Build history of the part. All positions in model axes, mm. A direction names the side the tool comes from. Give positions to 0.01 mm unless a question says otherwise; leave off trailing zeros. Order: outer loops, then holes, each group sorted by start corner. A loop starts at its lowest first (then second) coordinate and runs counter-clockwise, first axis right, second up. Notation, with made-up numbers: (39.25, 64) -> (77.25, 64) arc R37 cw to (77.25, 100) -> close; hole circle Ø10 at (73, 73.25). An arc over 180 degrees is marked (long way). Use a Markdown table: item, result. Add a question column.
```python
from build123d import *

# Parameters (mm, degrees)
F0_R     = 3.175
F0_W     = 44.45
F0_H     = 76.2
F0_R_2   = 1.5875
F1_DEPTH = 3.175


with BuildPart() as f1:
    # F0 (on Top) → F1 (new body)
    with BuildSketch(Plane.XY):
        with BuildLine():
            ThreePointArc((16.728534, 58.82596), (-5.496466, 81.05096), (-27.721466, 58.82596))
            Line((-27.721466, 58.82596), (16.728534, 58.82596))
        make_face()
        with Locations((-5.496466, 69.93846)):
            Circle(F0_R, mode=Mode.SUBTRACT)
        with Locations((-5.496466, 20.72596)):
            Rectangle(F0_W, F0_H)
        with Locations((-5.496466, -4.67404)):
            Circle(F0_R_2, mode=Mode.SUBTRACT)
        with Locations((-5.496466, 8.02596)):
            Circle(F0_R_2, mode=Mode.SUBTRACT)
        with BuildLine():
            Line((-22.562091, -9.75404), (-22.562091, 51.20596))
            ThreePointArc((-22.562091, 51.20596), (-18.196466, 55.571585), (-13.830841, 51.20596))
            Line((-13.830841, 51.20596), (-13.830841, -9.75404))
            ThreePointArc((-13.830841, -9.75404), (-18.196466, -14.119665), (-22.562091, -9.75404))
        make_face(mode=Mode.SUBTRACT)
        with Locations((-5.496466, 46.12596)):
            Circle(F0_R_2, mode=Mode.SUBTRACT)
        with Locations((-5.496466, 20.72596)):
            Circle(F0_R_2, mode=Mode.SUBTRACT)
        with Locations((-5.496466, 33.42596)):
            Circle(F0_R_2, mode=Mode.SUBTRACT)
        with BuildLine():
            Line((2.837909, -9.75404), (2.837909, 51.20596))
            ThreePointArc((2.837909, 51.20596), (7.203534, 55.571585), (11.569159, 51.20596))
            Line((11.569159, 51.20596), (11.569159, -9.75404))
            ThreePointArc((11.569159, -9.75404), (7.203534, -14.119665), (2.837909, -9.75404))
        make_face(mode=Mode.SUBTRACT)
        with BuildLine():
            Line((16.728534, -17.37404), (-27.721466, -17.37404))
            ThreePointArc((-27.721466, -17.37404), (-5.496466, -39.59904), (16.728534, -17.37404))
        make_face()
        with Locations((-5.496466, -28.48654)):
            Circle(F0_R, mode=Mode.SUBTRACT)
    extrude(amount=F1_DEPTH)


solid = f1.part
```
(1) Mould opens along Y. For faces 3 (the face through (-5.008, 81.046, 1.565)), 4 (the face through (-5.841, 44.576, 1.565)), 5 (the face through (-27.721, 20, 2)) say: released by +Y, released by -Y, zero draft, split by the parting line, or undercut.
(2) Tool access for faces 1 (the face through (-18.29, 55.57, 1.57)), 2 (the face through (-1, 22, 3.175)): list every direction of +Z, -Z, +X, -X, +Y, -Y with a clear straight run to the whole face (end or side of a thin tool).
(3) Band-saw the part on C-C on x = -21.5. Give the cut face in (y, z) (3 decimals), plus the area to 3 significant figures.
(4) Band-saw the part on A-A on x = -5.5. State how many separate pieces and enclosed holes the cut face has, plus the area to 3 significant figures.
(5) Wall check: probe 1 along X at (y, z) = (38, 2); probe 2 along Y at (x, z) = (-7.5, 1.55); probe 3 along Y at (x, z) = (-22, 1.65). Give the ranges that are in metal, low to high.
(6) Band-saw the part on B-B on y = 3. Give the cut face in (x, z) (3 decimals).
Response:
| question | item | result |
|---|---|---|
| 1 | face 3 | released by +Y |
| 1 | face 4 | undercut |
| 1 | face 5 | zero draft |
| 2 | face 1 | +Z, -Z |
| 2 | face 2 | +Z, +X, -X, +Y, -Y |
| 3 | outline | (-32.796, 0) -> (-12.608, 0) -> (-12.608, 3.175) -> (-32.796, 3.175) -> close; (54.06, 0) -> (74.248, 0) -> (74.248, 3.175) -> (54.06, 3.175) -> close |
| 3 | area | 128 mm² |
| 4 | separate pieces | 8 |
| 4 | enclosed holes | 0 |
| 4 | area | 292 mm² |
| 5 | probe 1 | x = -27.72 to -22.56, -13.83 to 2.84, 11.57 to 16.73 |
| 5 | probe 2 | y = -39.51 to -30.95, -26.02 to 67.48, 72.4 to 80.96 |
| 5 | probe 3 | y = -32.26 to -11.9, 53.35 to 73.71 |
| 6 | outline | (-27.721, 0) -> (-22.562, 0) -> (-22.562, 3.175) -> (-27.721, 3.175) -> close; (-13.831, 0) -> (2.838, 0) -> (2.838, 3.175) -> (-13.831, 3.175) -> close; (11.569, 0) -> (16.729, 0) -> (16.729, 3.175) -> (11.569, 3.175) -> close |
